Autodesk Inventor part; units mm, degrees
ref_plane "YZ Plane" through (0, 0, 0) normal (1, 0, 0) x (0, 1, 0)
ref_plane "XZ Plane" through (0, 0, 0) normal (0, 1, 0) x (-1, 0, 0)
ref_plane "XY Plane" through (0, 0, 0) normal (0, 0, 1) x (1, 0, 0)
sketch "Sketch1" plane through (0, 0, 0) normal (1, 0, 0) x (0, 1, 0)
  line L0 (0, 0) -> (0, 12.7)
  line L1 (0, 0) -> (-101.6, 0) construction
  arc A0 (-101.6, 0) -> (0, 0) centre (-50.8, 607.4796) ccw
  line L2 (-50.8, -2.1204) -> (-50.8, 0) construction
  line L3 (0, 12.7) -> (101.6, 12.7) construction
  arc A1 (0, 12.7) -> (101.6, 12.7) centre (50.8, 620.1796) ccw
  line L4 (-101.6, 0) -> (-101.6, 12.7)
  line L5 (-101.6, 12.7) -> (-203.2, 12.7) construction
  arc A2 (-203.2, 12.7) -> (-101.6, 12.7) centre (-152.4, 620.1796) ccw
  line L6 (17.3591, 11.4976) -> (17.3591, 36.923)
  line L7 (17.3591, 36.923) -> (-135.0409, 36.923)
  line L8 (-135.0409, 36.923) -> (-135.0409, 10.8269)
  dimension "d0" = 12.7
  dimension "d1" = 101.6
  dimension "d3" = 50.8
  dimension "d4" = 2.1204
  dimension "d5" = 609.6
  dimension "d6" = 101.6
  dimension "d7" = 609.6
  dimension "d8" = 12.7
  dimension "d9" = 101.6
  dimension "d10" = 609.6
  dimension "d11" = 152.4
  dimension "d12" = 25.4254
extrude "Extrusion1" add sketch "Sketch1" along normal mid plane 152.4
sketch "Sketch3" plane through (-76.2, -135.0409, 36.923) normal (0, 0, 1) x (1, 0, 0)
  line L0 (0, 0) -> (0, 152.4) construction
  line L1 (152.4, 152.4) -> (152.4, 0) construction
  line L2 (0, 152.4) -> (152.4, 0) construction
  line L3 (152.4, 0) -> (0, 0) construction
  line L4 (152.4, 135.0409) -> (152.4, 152.4) construction
  line L5 (0, 0) -> (152.4, 152.4) construction
  circle A0 centre (76.2, 76.2) radius 57.15
  line L6 (6.35, 6.35) -> (146.05, 6.35) construction
  line L7 (146.05, 6.35) -> (146.05, 146.05) construction
  line L8 (146.05, 146.05) -> (6.35, 146.05) construction
  line L9 (6.35, 146.05) -> (6.35, 6.35) construction
  line L10 (6.35, 6.35) -> (146.05, 146.05) construction
  line L11 (146.05, 6.35) -> (6.35, 146.05) construction
  line L12 (0, 152.4) -> (152.4, 152.4) construction
  point P0 (76.2, 135.0409)
  dimension "d15" = 114.3
  dimension "d16" = 6.35
  dimension "d17" = 6.35
extrude "Extrusion2" cut sketch "Sketch3" against normal through all
hole "Hole1" at (-69.85, 11.0091, 36.923) at (69.85, 11.0091, 36.923) at (69.85, -128.6909, 36.923) at (-69.85, -128.6909, 36.923) direction (0, 0, -1) diameter 5.1054 end through all
fillet "Fillet1" radius 6.35 4 edges at (-76.2, 17.3591, 24.2103) (76.2, 17.3591, 24.2103) (76.2, -135.0409, 23.8749) (-76.2, -135.0409, 23.8749)
equation "\"d0\" = sidingDepth"
equation "\"d1\" = sidingHeight"
equation "\"d5\" = radiusOfCurvature"
equation "\"d6\" = sidingHeight"
equation "\"d7\" = radiusOfCurvature"
equation "\"d11\" = outsideWidthOfVent"
equation "\"d13\" = outsideWidthOfVent"
equation "\"d15\" = ventHole"
equation "\"d27\" = ventRadius"
equation "\"sidingHeight\" = 101.6"
equation "\"sidingDepth\" = 12.7"
equation "\"radiusOfCurvature\" = 609.6"
equation "\"outsideWidthOfVent\" = 152.4"
equation "\"wallThicknessOfVent\" = 19.05"
equation "\"holeOffset\" = 6.35"
equation "\"ventHole\" = 114.3"
equation "\"ventRadius\" = 6.35"
properties part number "ventForDryer"
Input: part model. Units: mm. Frame: model coordinates. A direction names the side the tool comes from. Round coordinates to 2 decimals unless told otherwise and drop trailing zeros. Order: outer loops, then holes, each group sorted by start corner. A loop starts at its lowest first (then second) coordinate and runs counter-clockwise, first axis right, second up. Notation, with made-up numbers: (31.5, 83) - (56.5, 83) arc R32 cw to (56.5, 119) - close; hole circle Ø5 at (-4, 37.5). An arc over 180 degrees is marked (long way). Answer as a JSON object with one key per item and string values. Group by question number.
(1) Cut plane C-C (z = 24). Return loops of the section in (x, y), then the cut area to 3 significant figures.
(2) Cut plane D-D (y = -70.5). Return loops of the section in (x, z), then the cut area to 3 significant figures.
(3) Pin query (flat end, axial travel): P1, Ø4, axis at x = -49.5, z = 6, coming from the -Y side; P2, Ø4, axis at x = 69.85, y = -128.69, coming from the +Z side; P3, Ø6.5, axis at x = 14.5, z = 5, coming from the +Y side. Return the tip coordinate at first contact, or that it passes through.
(4) Material intervals for probe 1 along Y at (x, z) = (69.85, 22.25); probe 2 along Y at (x, z) = (68, 27.5); probe 3 along Y at (x, z) = (0, 26), sorted ascending. Write a range as from..to.
(5) Cut plane A-A (x = -20.5). Return loops of the section in (y, z).
(6) Reachability of faces 1 (the face through (67.32, 11.34, 24.14)), 2 (the face through (-1.07, 8.8, 12.03)) from +Z, -Z, +X, -X, +Y, -Y: full face, straight path, thin tool, end or side. Return the list, or none.
(7) Cut plane B-B (y = -42). Return loops of the section in (x, z), then the cut area to 3 significant figures.
(8) Draft query along Y for faces 3 (the face through (74.39, 15.45, 24.39)), 4 (the face through (-1, -135.041, 24)), 5 (the face through (68.125, -126.809, 23.753)). Return one class per face: released by +Y, released by -Y, zero draft, split by the parting line, or undercut.
Here are the results:
{
 "1": {"outline": "(-76.2, -128.69) arc R6.35 ccw to (-69.85, -135.04) - (69.85, -135.04) arc R6.35 ccw to (76.2, -128.69) - (76.2, 11.01) arc R6.35 ccw to (69.85, 17.36) - (-69.85, 17.36) arc R6.35 ccw to (-76.2, 11.01) - close; hole circle Ø5.11 at (-69.85, -128.69); hole circle Ø5.11 at (-69.85, 11.01); hole circle Ø114.3 at (0, -58.84); hole circle Ø5.11 at (69.85, -128.69); hole circle Ø5.11 at (69.85, 11.01)", "area": "12,800 mm^2"},
 "2": {"outline": "(-76.2, -1.8) - (-55.95, -1.8) - (-55.95, 36.92) - (-76.2, 36.92) - close; (55.95, -1.8) - (76.2, -1.8) - (76.2, 36.92) - (55.95, 36.92) - close", "area": "1,570 mm^2"},
 "3": {"P1": "stops at y = -101.6", "P2": "passes through", "P3": "stops at y = 0"},
 "4": {"probe 1": "y = -135.04..-131.24, -126.14..8.46, 13.56..17.36", "probe 2": "y = -135.04..-130.45, -126.93..9.25, 12.77..17.36", "probe 3": "y = -135.04..-115.99, -1.69..17.36"},
 "5": {"outline": "(-135.04, 10.83) arc R609.6 ccw to (-112.19, 11.91) - (-112.19, 36.92) - (-135.04, 36.92) - close; (-5.49, -0.43) arc R609.6 ccw to (0, 0) - (0, 12.7) arc R609.6 ccw to (17.36, 11.5) - (17.36, 36.92) - (-5.49, 36.92) - close"},
 "6": {"face 1": "+Z, -Z", "face 2": "-Z, +X, -X"},
 "7": {"outline": "(-76.2, -2.06) - (-54.61, -2.06) - (-54.61, 36.92) - (-76.2, 36.92) - close; (54.61, -2.06) - (76.2, -2.06) - (76.2, 36.92) - (54.61, 36.92) - close", "area": "1,680 mm^2"},
 "8": {"face 3": "released by +Y", "face 4": "released by -Y", "face 5": "undercut"}
}
